Model file for the job. Use its own axes, mm. Face numbers are marked on the shaded views. A direction names the side the tool comes from. Give positions to 0.01 mm unless a question says otherwise; leave off trailing zeros. Write each loop counter-clockwise with the first axis right and the second up, starting at its lowest first coordinate (ties: lowest second). Pieces come first, ordered by that corner, then holes. Notation, with made-up numbers: (-9.5, -7.5) - (14.5, -7.5) arc R35 cw to (14.5, 30.5) - close; hole circle Ø2 at (36, 30). An arc over 180 degrees is marked (long way). One line per item, written item: value. Start each with the question number.
(1) Cut at A-A, the plane z = -12. List the corners of the cut face in (x, y).
(2) Cut at B-B, the plane x = 3.5. List the corners of the cut face in (y, z), and give its area (3 significant figures).
(3) Mould opens along Z. For the marked faces 1, 2, 3 and 4 say: pulls with the +Z half, pulls with the -Z half, needs draft (parallel to the pull), parting line crosses it, or undercut.
(4) Drop flat-ended pins along their axis: P1, Ø6, axis at x = 10, y = 13, coming from the -Z side; P2, Ø1.5, axis at x = 13.5, z = -5.5, coming from the -Y side. Give the stop position or say it passes through.
(5) 3-axis set-ups, long thin cutter, end or side, ignore diameter. For the marked faces 5 and 6: which of +Z, -Z, +X, -X, +Y, -Y reach the whole face in a straight line?
(6) Cut at C-C, the plane y = 12.5. List the corners of the cut face in (x, z), and give its area (3 significant figures).
(7) Probe L1, parallel to X at y = 12, z = 5.5; L2, parallel to Z at x = 12, y = 18; L3, parallel to Y at x = 6.5, z = 12.5. List the from-to ranges inside material, lowest first.
from build123d import *

# Parameters (mm, degrees)
SKETCH1_W           = 65.7
SKETCH1_H           = 30.2
SKETCH1_W_2         = 64.5
SKETCH1_H_2         = 29
BOSS_EXTRUDE1_DEPTH = 22
SKETCH2_W           = 65.7
SKETCH2_H           = 30.2
BOSS_EXTRUDE2_DEPTH = 0.6
SKETCH3_W           = 60
SKETCH3_H           = 15
CUT_EXTRUDE1_DEPTH  = 10.6
CHAMFER1_SIZE       = 1.5


with BuildPart() as part:
    # Sketch1 → Boss-Extrude1 (new body)
    with BuildSketch(Plane(origin=(0, 0, 0), x_dir=(1, 0, 0), z_dir=(0, 1, 0))):
        Rectangle(SKETCH1_W, SKETCH1_H)
        Rectangle(SKETCH1_W_2, SKETCH1_H_2, mode=Mode.SUBTRACT)
    extrude(amount=BOSS_EXTRUDE1_DEPTH)

    # Sketch2 → Boss-Extrude2 (add)
    with BuildSketch(Plane(origin=(0, 22, 0), x_dir=(1, 0, 0), z_dir=(0, 1, 0))):
        Rectangle(SKETCH2_W, SKETCH2_H)
    extrude(amount=BOSS_EXTRUDE2_DEPTH)

    # Sketch3 → Cut-Extrude1 (cut)
    with BuildSketch(Plane(origin=(0, 0, -15.1), x_dir=(-1, 0, 0), z_dir=(0, 0, -1))):
        with Locations((0, 7.5)):
            Rectangle(SKETCH3_W, SKETCH3_H)
    extrude(amount=-CUT_EXTRUDE1_DEPTH, mode=Mode.SUBTRACT)

    # Chamfer1
    chamfer1_edges = [part.edges().sort_by_distance(p)[0] for p in [
        (32.25, 11, 14.5),
        (32.25, 11, -14.5),
        (-32.25, 11, -14.5),
        (-32.25, 11, 14.5),
        (32.25, 22, 0),
        (0, 22, -14.5),
        (-32.25, 22, 0),
        (0, 22, 14.5),
    ]]
    chamfer(chamfer1_edges, length=CHAMFER1_SIZE)


solid = part.part
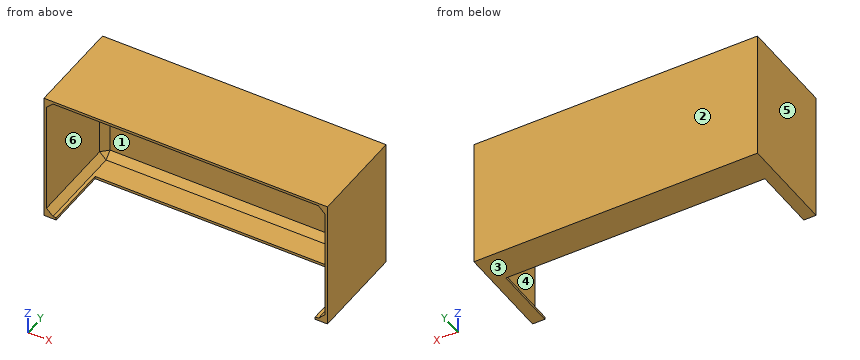
Answers follow:
1. outline: (-32.85, 0) - (-32.25, 0) - (-32.25, 20.5) - (-30.75, 22) - (30.75, 22) - (32.25, 20.5) - (32.25, 0) - (32.85, 0) - (32.85, 22.6) - (-32.85, 22.6) - close
2. outline: (0, 14.5) - (20.5, 14.5) - (22, 13) - (22, -13) - (20.5, -14.5) - (15, -14.5) - (15, -15.1) - (22.6, -15.1) - (22.6, 15.1) - (0, 15.1) - close
2. area: 37.8 mm²
3. face 1: undercut
3. face 2: needs draft
3. face 3: pulls with the -Z half
3. face 4: undercut
4. P1: stops at z = -15.1
4. P2: stops at y = 22
5. face 5: +Z, -Z, -X, +Y, -Y
5. face 6: -Y
6. outline: (-32.85, -15.1) - (-30, -15.1) - (-30, -14.5) - (-30.75, -14.5) - (-32.25, -13) - (-32.25, 13) - (-30.75, 14.5) - (30.75, 14.5) - (32.25, 13) - (32.25, -13) - (30.75, -14.5) - (30, -14.5) - (30, -15.1) - (32.85, -15.1) - (32.85, 15.1) - (-32.85, 15.1) - close
6. area: 82.1 mm²
7. L1: x = -32.85 to -32.25, 32.25 to 32.85
7. L2: z = -15.1 to -14.5, 14.5 to 15.1
7. L3: y = 22 to 22.6
